```python
from build123d import *

# Parameters (mm, degrees)
F1_DEPTH = 25.4
F3_DEPTH = 19.05


with BuildPart() as f1:
    # F0 (on Front) → F1 (new body)
    with BuildSketch(Plane.XZ):
        Polygon((21.997045, 38.1), (0, 0), (457.2, 0), (435.202955, 38.1), align=None)
    extrude(amount=F1_DEPTH)

    # F2 (on face) → F3 (cut)
    with BuildSketch(Plane.XY.offset(38.1)):
        Polygon((233.861157, 0), (197.940133, 0), (223.340133, -25.4), (259.261157, -25.4), align=None)
    extrude(amount=-F3_DEPTH, mode=Mode.SUBTRACT)


solid = f1.part
```
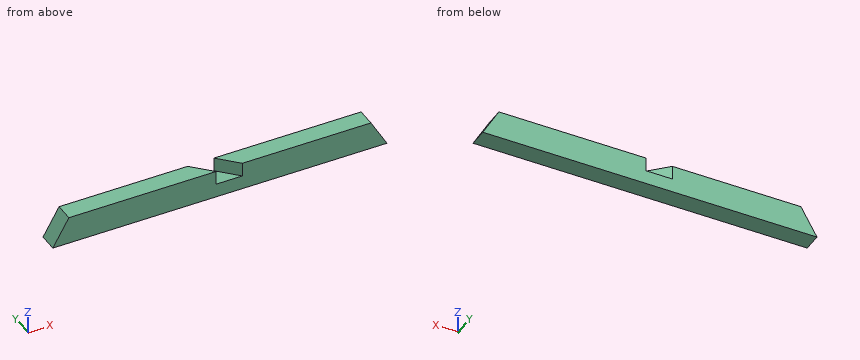
Check sheet for the modelled part. Datum: model origin and axes. Units: mm. Coordinates: 2 decimals unless noted, no trailing zeros. Loops run counter-clockwise (first coordinate to the right, second up) from the corner with the lowest first, then second, coordinate; pieces in that order, holes last.
1) Material ranges on probe 1 along X at (y, z) = (-6, 35); probe 2 along X at (y, z) = (-10.25, 28.5); probe 3 along Z at (x, y) = (243, -18.25), recorded low to high.
2) Gauge pin test, flat ends, axial feed: pin 1 (10 mm diameter, centred on y = -14.5, z = 8, fed in from -X); pin 2 (6 mm diameter, centred on y = -20.5, z = 6.5, fed in from -X); pin 3 (1.5 mm diameter, centred on y = -5.5, z = 5, fed in from +X). Record the tip position at first contact, or that the pin passes through.
3) Sectioned sample at A-A (z = 32). Record the boundary of the cut face in (x, y).
4) Sectioned sample at B-B (y = -14.25). Record the boundary of the cut face in (x, z), and give its area (3 significant figures).
Check sheet entries:
1. probe 1: x = 20.21 to 203.94, 239.86 to 436.99
1. probe 2: x = 16.45 to 208.19, 244.11 to 440.75
1. probe 3: z = 0 to 19.05
2. pin 1: stops at x = 1.73
2. pin 2: stops at x = 2.02
2. pin 3: stops at x = 454.75
3. outline: (18.48, -25.4) - (223.34, -25.4) - (197.94, 0) - (18.48, 0) - close; (233.86, 0) - (259.26, -25.4) - (438.72, -25.4) - (438.72, 0) - close
4. outline: (0, 0) - (457.2, 0) - (435.2, 38.1) - (248.11, 38.1) - (248.11, 19.05) - (212.19, 19.05) - (212.19, 38.1) - (22, 38.1) - close
4. area: 15,900 mm2
